```python
from build123d import *

# Parameters (mm, degrees)
SKETCH1_R                  = 200
BOSS_EXTRUDE1_DEPTH        = 50
SKETCH2_R                  = 15
SKETCH2_R_2                = 30
CUT_EXTRUDE1_DEPTH         = 15
M12X1_5_TAPPED_HOLE1_D     = 10.5
M12X1_5_TAPPED_HOLE1_DEPTH = 25.34548175
M12X1_5_TAPPED_HOLE1_TIP   = 3.15451825
CIRPATTERN5_COUNT          = 3
CIRPATTERN5_ANGLE          = 180
CIRPATTERN6_COUNT          = 4
M12X1_5_TAPPED_HOLE2_D     = 10.5
M12X1_5_TAPPED_HOLE2_DEPTH = 25.34548175
M12X1_5_TAPPED_HOLE2_TIP   = 3.15451825
SKETCH3_W                  = 30
SKETCH3_H                  = 60
CUT_EXTRUDE2_DEPTH         = 15
M6_TAPPED_HOLE3_D          = 5
M6_TAPPED_HOLE3_DEPTH      = 13.497848452
M6_TAPPED_HOLE3_TIP        = 1.502151548
SKETCH32_R                 = 3
CUT_EXTRUDE3_DEPTH         = 15
M12X1_5_TAPPED_HOLE3_D     = 10.5
M12X1_5_TAPPED_HOLE3_DEPTH = 25.34548175
M12X1_5_TAPPED_HOLE3_TIP   = 3.15451825


with BuildPart() as part:
    # Sketch1 → Boss-Extrude1 (new body)
    with BuildSketch(Plane(origin=(0, 0, 0), x_dir=(1, 0, 0), z_dir=(0, 1, 0))):
        Circle(SKETCH1_R)
    extrude(amount=BOSS_EXTRUDE1_DEPTH)

    # Sketch2 → Cut-Extrude1 (cut)
    with BuildSketch(Plane(origin=(0, 50, 0), x_dir=(1, 0, 0), z_dir=(0, 1, 0))):
        with Locations((0, -69.113872591)):
            Circle(SKETCH2_R)
        with Locations((25.69461295, 46.354666069)):
            Circle(SKETCH2_R)
        with Locations((-42.327685627, 31.896492385)):
            Circle(SKETCH2_R_2)
        with BuildLine():
            Line((31.001143439, -33.886276935), (72.945217779, -60.052947106))
            ThreePointArc((72.945217779, -60.052947106), (76.850049502, -7.09303501), (31.001143439, -33.886276935))
        make_face()
    extrude(amount=-CUT_EXTRUDE1_DEPTH, mode=Mode.SUBTRACT)

    # M12x1.5 Tapped Hole1
    with Locations(Plane(origin=(0, 35, 0), x_dir=(1, 0, 0), z_dir=(0, 1, 0))):
        with Locations((25.69461295, 46.354666069), (0, -69.113872591)):
            Hole(M12X1_5_TAPPED_HOLE1_D / 2, depth=M12X1_5_TAPPED_HOLE1_DEPTH)
            with Locations((0, 0, -(M12X1_5_TAPPED_HOLE1_DEPTH + M12X1_5_TAPPED_HOLE1_TIP / 2))):  # 118° drill point
                Cone(0, M12X1_5_TAPPED_HOLE1_D / 2, M12X1_5_TAPPED_HOLE1_TIP, mode=Mode.SUBTRACT)

    # Sketch18 → M6 Tapped Hole1 (revolve, cut)
    with BuildSketch(Plane(origin=(44.002440842, 35, 21.960267616), x_dir=(0, 0, 1), z_dir=(1, 0, 0))):
        Polygon((0, 0), (0, 15), (2.5, 13.497848452), (2.5, 0), align=None)
    m6_tapped_hole1 = revolve(axis=Axis((44.002440842, 41.35, 21.960267616), (0, -1, 0)), mode=Mode.SUBTRACT)

    # CirPattern5: M6 Tapped Hole1 ×3 about axis
    cirpattern5_axis = Axis((60.971197017, 0, 32.546169272), (0, -1, 0))
    for i in range(1, CIRPATTERN5_COUNT):
        add(m6_tapped_hole1.rotate(cirpattern5_axis, i * CIRPATTERN5_ANGLE / (CIRPATTERN5_COUNT - 1)), mode=Mode.SUBTRACT)

    # Sketch21 → M6 Tapped Hole2 (revolve, cut)
    with BuildSketch(Plane(origin=(-42.327685627, 35, -51.896492385), x_dir=(0, 0, 1), z_dir=(1, 0, 0))):
        Polygon((0, 0), (0, 15), (2.5, 13.497848452), (2.5, 0), align=None)
    m6_tapped_hole2 = revolve(axis=Axis((-42.327685627, 41.35, -51.896492385), (0, -1, 0)), mode=Mode.SUBTRACT)

    # CirPattern6: M6 Tapped Hole2 ×4 about axis
    cirpattern6_axis = Axis((-42.327685627, 0, -31.896492385), (0, 1, 0))
    for i in range(1, CIRPATTERN6_COUNT):
        add(m6_tapped_hole2.rotate(cirpattern6_axis, i * 360 / CIRPATTERN6_COUNT), mode=Mode.SUBTRACT)

    # M12x1.5 Tapped Hole2
    with Locations(Plane(origin=(0, 50, 0), x_dir=(1, 0, 0), z_dir=(0, 1, 0))):
        with Locations((-0.014790744, 0.024833856)):
            Hole(M12X1_5_TAPPED_HOLE2_D / 2, depth=M12X1_5_TAPPED_HOLE2_DEPTH)
            with Locations((0, 0, -(M12X1_5_TAPPED_HOLE2_DEPTH + M12X1_5_TAPPED_HOLE2_TIP / 2))):  # 118° drill point
                Cone(0, M12X1_5_TAPPED_HOLE2_D / 2, M12X1_5_TAPPED_HOLE2_TIP, mode=Mode.SUBTRACT)

    # Sketch3 → Cut-Extrude2 (cut)
    with BuildSketch(Plane(origin=(0, 50, 0), x_dir=(1, 0, 0), z_dir=(0, 1, 0))):
        with Locations((58.112318667, -137.113872591)):
            Rectangle(SKETCH3_W, SKETCH3_H)
        Polygon((110.814391162, 111.220861865), (81.72598544, 58.743584377), (107.964624184, 44.199381516), (137.053029906, 96.676659004), align=None)
        with Locations((-100.327685627, 99.896492385)):
            Rectangle(SKETCH3_W, SKETCH3_H)
        with Locations((-57.887681333, -137.113872591)):
            Rectangle(SKETCH3_W, SKETCH3_H)
        Polygon((9.358321352, 167.458446261), (35.596960096, 152.9142434), (10.672314373, 107.948645684), (10.672314373, 99.896492385), (30.672314373, 99.896492385), (30.672314373, 69.896492385), (0.672314373, 69.896492385), (0.672314373, 129.896492385), (10.672314373, 129.896492385), (11.746380439, 131.834173793), (-5.185881509, 141.219807517), align=None)
    extrude(amount=-CUT_EXTRUDE2_DEPTH, mode=Mode.SUBTRACT)

    # M6 Tapped Hole3
    with Locations(Plane(origin=(0, 35, 0), x_dir=(1, 0, 0), z_dir=(0, 1, 0))):
        with Locations((123.458749371, 92.77851371), (104.06647889, 57.793662051), (-105.327685627, 119.896492385), (-105.327685627, 79.896492385), (-62.887681333, -117.113872591), (-62.887681333, -157.113872591), (63.112318667, -117.113872591), (63.112318667, -157.113872591), (13.256466646, 153.864165726), (20.672314373, 79.896492385)):
            Hole(M6_TAPPED_HOLE3_D / 2, depth=M6_TAPPED_HOLE3_DEPTH)
            with Locations((0, 0, -(M6_TAPPED_HOLE3_DEPTH + M6_TAPPED_HOLE3_TIP / 2))):  # 118° drill point
                Cone(0, M6_TAPPED_HOLE3_D / 2, M6_TAPPED_HOLE3_TIP, mode=Mode.SUBTRACT)

    # Sketch32 → Cut-Extrude3 (cut)
    with BuildSketch(Plane(origin=(0, 35, 0), x_dir=(1, 0, 0), z_dir=(0, 1, 0))):
        with Locations((56.457837304, -13.062083867)):
            Circle(SKETCH32_R)
    extrude(amount=-CUT_EXTRUDE3_DEPTH, mode=Mode.SUBTRACT)

    # M12x1.5 Tapped Hole3
    with Locations(Plane(origin=(0, 50, 0), x_dir=(1, 0, 0), z_dir=(0, 1, 0))):
        with Locations((35.989041426, -60.006192032)):
            Hole(M12X1_5_TAPPED_HOLE3_D / 2, depth=M12X1_5_TAPPED_HOLE3_DEPTH)
            with Locations((0, 0, -(M12X1_5_TAPPED_HOLE3_DEPTH + M12X1_5_TAPPED_HOLE3_TIP / 2))):  # 118° drill point
                Cone(0, M12X1_5_TAPPED_HOLE3_D / 2, M12X1_5_TAPPED_HOLE3_TIP, mode=Mode.SUBTRACT)


solid = part.part
```
For this review, take the finished solid that the model builds, in its own axes (mm). Round coordinates to 2 decimals unless told otherwise and drop trailing zeros. Write each loop counter-clockwise with the first axis right and the second up, starting at its lowest first coordinate (ties: lowest second). Pieces come first, ordered by that corner, then holes. Notation, with made-up numbers: (57, 65.25) -> (69, 65.25) arc R15 ccw to (69, 80.25) -> close; hole circle Ø9 at (77, 16.5). An arc over 180 degrees is marked (long way). Use one line per item in the form item = value.
Q1. Clearance check with flat-ended pins moving along their axes: pin 1 Ø7.5 at (y, z) = (39.5, 131.5) entering from +X; pin 2 Ø10 at (y, z) = (10, -80.5) entering from -X; pin 3 Ø8.5 at (x, z) = (-0.01, -0.02) entering from +Y. State where each tip first meets the part, or that it passes through.
Resolved:
pin_1 = 153.88
pin_2 = -185.2
pin_3 = 24.06
Q2. The part is to be moulded in two halves that separate along X. For faces 1 (the cylindrical face through (190.764, 24.65, -60.075)), 2 (the flat face through (-43, 35, -32)), 3 (the flat face through (-3, 0, -3)), say which applies: released by +X, released by -X, zero draft, split by the parting line, or undercut.
Resolved:
face_1 = split by the parting line
face_2 = undercut
face_3 = zero draft
Q3. Consider section A-A (y = 30). State how many separate pieces and enclosed holes the cut face has, then the cut area to 3 significant figures.
Resolved:
separate_pieces = 1
enclosed_holes = 22
area = 125,000 mm²
Q4. Consider section C-C (x = -156.5). State the section outline as (y, z) points, then the cut area to 3 significant figures.
Resolved:
outline = (0, -124.53) -> (50, -124.53) -> (50, 124.53) -> (0, 124.53) -> close
area = 12,500 mm²
Q5. Consider section B-B (z = 79.5). State the section outline as (x, y) points, then the cut area to 3 significant figures.
Resolved:
outline = (-183.52, 0) -> (183.52, 0) -> (183.52, 50) -> (10.82, 50) -> (10.82, 35) -> (-10.82, 35) -> (-10.82, 50) -> (-183.52, 50) -> close
area = 18,000 mm²
Q6. To check wall thickness, follow probe 1 along Y at (x, z) = (25.5, -34); probe 2 along X at (y, z) = (11, 3); probe 3 along X at (y, z) = (37, 19.5). State the ranges of each line that lie inside material, in increasing order. Write a range as from..to.
Resolved:
probe_1 = 0..35
probe_2 = -199.98..199.98
probe_3 = -199.05..33.96, 87.99..199.05
